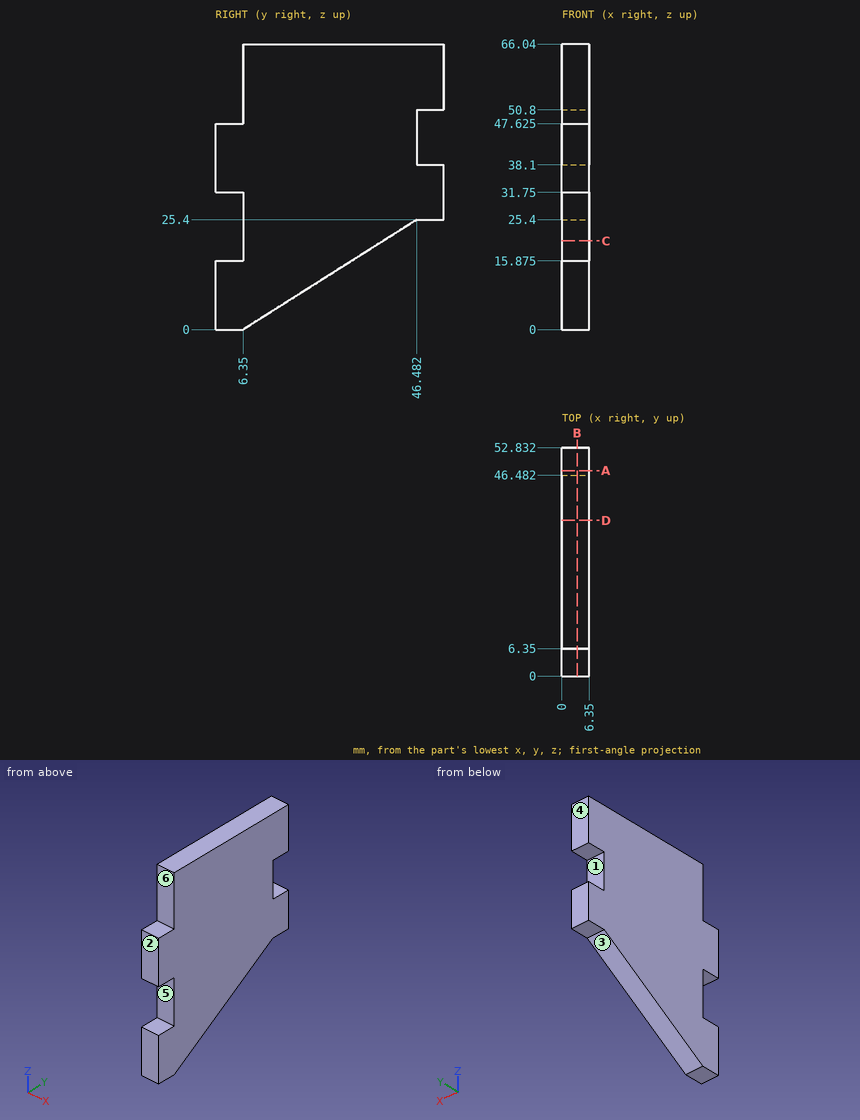
Check sheet for the drawn part. Datum: minimum x, y, z corner. Units: mm. A direction names the side the tool comes from. Round coordinates to 2 decimals unless told otherwise and drop trailing zeros. Loops run counter-clockwise (first coordinate to the right, second up) from the corner with the lowest first, then second, coordinate; pieces in that order, holes last.
Item 1: Thickness scan on line 1 (Z direction, x = 3.75, y = 51); line 2 (Y direction, x = 1.5, z = 46.5); line 3 (Z direction, x = 1, y = 5) (3 decimals). Record the ranges inside material, lowest first.
Item 2: Mould release check, pull along Z, two halves, no side actions. Record for the marked faces 1, 2 and 3: pulls with the +Z half, pulls with the -Z half, needs draft (parallel to the pull), parting line crosses it, or undercut.
Item 3: Cross-section at C-C on z = 20.5. Record the boundary of the cut face in (x, y).
Item 4: Cross-section at D-D on y = 36. Record the boundary of the cut face in (x, z), then the cut area to 3 significant figures.
Item 5: Access from +Z, -Z, +X, -X, +Y, -Y to the whole of each face (thin tool, end or side, straight path). Record for the marked faces 4, 5 and 6.
Item 6: Cross-section at A-A on y = 47.5. Record the boundary of the cut face in (x, z).
Item 7: Cross-section at B-B on x = 3.5. Record the boundary of the cut face in (y, z) (3 decimals).
Item 8: Gauge pin test, flat ends, axial feed: pin 1 (3 mm diameter, centred on x = 2.5, z = 20, fed in from -Y); pin 2 (3 mm diameter, centred on x = 2, y = 4, fed in from +Z) (3 decimals); pin 3 (3 mm diameter, centred on x = 5, y = 14.5, fed in from -Z). Record the tip position at first contact, or that the pin passes through.
Answer sheet:
1. line 1: z = 25.4 to 38.1, 50.8 to 66.04
1. line 2: y = 0 to 46.48
1. line 3: z = 0 to 15.875, 31.75 to 47.625
2. face 1: undercut
2. face 2: needs draft
2. face 3: pulls with the -Z half
3. outline: (0, 6.35) - (6.35, 6.35) - (6.35, 38.74) - (0, 38.74) - close
4. outline: (0, 18.77) - (6.35, 18.77) - (6.35, 66.04) - (0, 66.04) - close
4. area: 300 mm2
5. face 4: +Z, -Z, +X, -X, +Y
5. face 5: +X, -X, -Y
5. face 6: +Z, +X, -X, -Y
6. outline: (0, 25.4) - (6.35, 25.4) - (6.35, 38.1) - (0, 38.1) - close; (0, 50.8) - (6.35, 50.8) - (6.35, 66.04) - (0, 66.04) - close
7. outline: (0, 0) - (6.35, 0) - (46.482, 25.4) - (52.832, 25.4) - (52.832, 38.1) - (46.482, 38.1) - (46.482, 50.8) - (52.832, 50.8) - (52.832, 66.04) - (6.35, 66.04) - (6.35, 47.625) - (0, 47.625) - (0, 31.75) - (6.35, 31.75) - (6.35, 15.875) - (0, 15.875) - close
8. pin 1: stops at y = 6.35
8. pin 2: stops at z = 47.625
8. pin 3: stops at z = 4.21
